Geometry: final body of the model. Coordinates: model frame, mm. A direction names the side the tool comes from. Round coordinates to 2 decimals unless told otherwise and drop trailing zeros. Loops run counter-clockwise (first coordinate to the right, second up) from the corner with the lowest first, then second, coordinate; pieces in that order, holes last. Notation, with made-up numbers: (-22, 8) - (5, 8) arc R9 cw to (5, 23) - close; hole circle Ø7 at (76.5, -4). An arc over 180 degrees is marked (long way). Answer as CSV lines item,"result".
from build123d import *

# Parameters (mm, degrees)
SKETCH_W     = 29
SKETCH_H     = 10
SKETCH_R     = 2.1
PAD_DEPTH    = 10
SKETCH001_R  = 7.6
POCKET_DEPTH = 10.001


with BuildPart() as part:
    # Sketch → Pad (new body)
    with BuildSketch(Plane(origin=(-52.3, -59.3, 36), x_dir=(1, 0, 0), z_dir=(0, -1, 0))):
        with Locations((-22.630757, 6.507574)):
            Rectangle(SKETCH_W, SKETCH_H)
        with Locations((-34.130757, 6.507574)):
            Circle(SKETCH_R, mode=Mode.SUBTRACT)
        with Locations((-11.130757, 6.507574)):
            Circle(SKETCH_R, mode=Mode.SUBTRACT)
    extrude(amount=PAD_DEPTH)

    # Sketch001 → Pocket (cut, through all)
    with BuildSketch(Plane(origin=(-52.3, -59.3, 37.507574), x_dir=(1, 0, 0), z_dir=(0, 0, -1))):
        with Locations((-22.630757, 10.5)):
            Circle(SKETCH001_R)
        Polygon((-8.130757, 7), (-13.130757, 7), (-18.130757, 2), (-27.130757, 2), (-32.130757, 7), (-37.130757, 7), (-37.130757, 0), (-8.130757, 0), align=None)
    extrude(amount=-POCKET_DEPTH, mode=Mode.SUBTRACT)


solid = part.part
(1) Section C-C (y = -63.25). Output: boundary loops of the cut face in (x, z).
Findings below:
outline,"(-81.38, 37.51) - (-78.79, 37.51) - (-78.79, 47.51) - (-81.38, 47.51) - close; (-71.08, 37.51) - (-68.48, 37.51) - (-68.48, 47.51) - (-71.08, 47.51) - close"
(2) Section A-A (y = -67.75). Output: boundary loops of the cut face in (x, z).
Findings below:
outline,"(-89.43, 37.51) - (-82.25, 37.51) - (-82.25, 47.51) - (-89.43, 47.51) - close; (-67.61, 37.51) - (-60.43, 37.51) - (-60.43, 47.51) - (-67.61, 47.51) - close; hole circle Ø4.2 at (-86.43, 42.51); hole circle Ø4.2 at (-63.43, 42.51)"
(3) Section D-D (z = 43.75). Output: boundary loops of the cut face in (x, y), and give its area (3 significant figures).
Findings below:
outline,"(-89.43, -69.3) - (-88.12, -69.3) - (-88.12, -66.3) - (-89.43, -66.3) - close; (-84.74, -69.3) - (-82.51, -69.3) arc R7.6 cw to (-67.35, -69.3) - (-65.12, -69.3) - (-65.12, -66.3) - (-65.43, -66.3) - (-70.43, -61.3) - (-79.43, -61.3) - (-84.43, -66.3) - (-84.74, -66.3) - close; (-61.74, -69.3) - (-60.43, -69.3) - (-60.43, -66.3) - (-61.74, -66.3) - close"
area,"53.5 mm2"
(4) Section B-B (z = 46.5). Output: boundary loops of the cut face in (x, y), and give its area (3 significant figures).
Findings below:
outline,"(-89.43, -69.3) - (-82.51, -69.3) arc R7.6 cw to (-67.35, -69.3) - (-60.43, -69.3) - (-60.43, -66.3) - (-65.43, -66.3) - (-70.43, -61.3) - (-79.43, -61.3) - (-84.43, -66.3) - (-89.43, -66.3) - close"
area,"73.9 mm2"
(5) Pin query (flat end, axial travel): P1, Ø1.5, axis at y = -65.5, z = 43.5, coming from the +X side; P2, Ø2, axis at x = -70.5, y = -67.5, coming from the -Z side; P3, Ø1.5, axis at x = -86.5, z = 44, coming from the +Y side; P4, Ø5, axis at x = -86.43, z = 42.51, coming from the +Y side. Return the tip coordinate at first contact, or that it passes through.
Findings below:
P1,"x = -65.48"
P2,"through"
P3,"y = -66.3"
P4,"y = -65.8"
(6) Draft query along X for faces 1 (the face through (-60.431, -68, 42)), 2 (the face through (-65.5, -69.3, 43.7)), 3 (the face through (-86.7, -67.73, 44.59)). Return one class per face: pulls with the +X half, pulls with the -X half, needs draft (parallel to the pull), parting line crosses it, or undercut.
Findings below:
face 1,"pulls with the +X half"
face 2,"needs draft"
face 3,"undercut"
(7) Material intervals for line 1 along X through (y, z) = (-66.5, 42); line 2 along Y through (x, z) = (-65, 38.5); line 3 along X through (y, z) = (-63, 39.5), sorted ascending.
Findings below:
line 1,"-89.43 to -88.47, -84.39 to -81.78, -68.08 to -65.47, -61.39 to -60.43"
line 2,"-69.3 to -66.3"
line 3,"-81.13 to -78.32, -71.54 to -68.73"
(8) Access query for faces 4 (the face through (-61, -66.3, 42)), 5 (the face through (-84, -69.3, 44)), 6 (the face through (-89, -66.3, 42)). Directions: +Z, -Z, +X, -X, +Y, -Y. A direction counts if a zero-diameter tool reaches every point of the face in a straight line with its end or side. Return the directions, or none.
Findings below:
face 4,"+Z, -Z, +X, +Y"
face 5,"+Z, -Z, +X, -X, -Y"
face 6,"+Z, -Z, -X, +Y"
